Verification items for the finished model (mm, model axes). Face numbers are marked on the shaded views. Give positions to 0.01 mm unless a question says otherwise; leave off trailing zeros. Order: outer loops, then holes, each group sorted by start corner. A loop starts at its lowest first (then second) coordinate and runs counter-clockwise, first axis right, second up. Notation, with made-up numbers: (-20, 63.5) - (0, 63.5) arc R8 ccw to (0, 72.5) - close; hole circle Ø8 at (32.25, 38.5). An arc over 180 degrees is marked (long way). Answer as a JSON object with one key per item and string values.
```python
from build123d import *

# Parameters (mm, degrees)
SKETCH_1_R      = 30
EXTRUDE_1_DEPTH = 32
FILLET_1_R      = 10
SKETCH_2_R      = 5
EXTRUDE_2_DEPTH = 12


with BuildPart() as part:
    # Эскиз1 → Бобышка-Вытянуть1 (new body)
    with BuildSketch(Plane.XY):
        Circle(SKETCH_1_R)
    extrude(amount=EXTRUDE_1_DEPTH)

    # Скругление1
    fillet_1_edges = [part.edges().sort_by_distance(p)[0] for p in [
        (-30, 0, 0),
        (-30, 0, 32),
    ]]
    fillet(fillet_1_edges, radius=FILLET_1_R)

    # Эскиз2 → Бобышка-Вытянуть2 (add)
    with BuildSketch(Plane(origin=(0, 0, 0), x_dir=(-1, 0, 0), z_dir=(0, 0, -1))):
        with Locations(Location((0, 0, 0), (0, 0, 180))):
            Circle(SKETCH_2_R)
        with BuildLine():
            Line((-1.198957881, 2.75), (1.198957881, 2.75))
            ThreePointArc((1.198957881, 2.75), (3, 0), (1.198957881, -2.75))
            Line((1.198957881, -2.75), (-1.198957881, -2.75))
            ThreePointArc((-1.198957881, -2.75), (-3, 0), (-1.198957881, 2.75))
        make_face(mode=Mode.SUBTRACT)
    extrude(amount=EXTRUDE_2_DEPTH)


solid = part.part
```
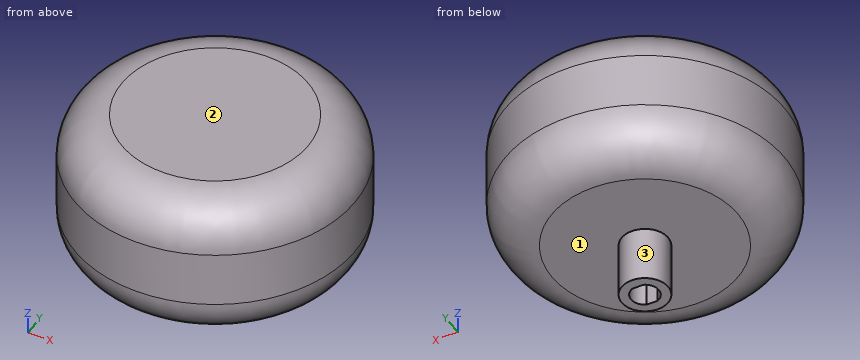
(1) Gauge pin test, flat ends, axial feed: pin 1 Ø1.2 at (x, z) = (-0.5, -4) entering from +Y; pin 2 Ø1 at (y, z) = (17.5, 7) entering from -X; pin 3 Ø6 at (y, z) = (22, 1) entering from +X. Record the tip position at first contact, or that the pin passes through.
Computed values:
{"pin 1": "stops at y = 5", "pin 2": "stops at x = -24.2", "pin 3": "stops at x = 18.68"}
(2) Section check A-A (y = 0). Record the cut outline in (x, z).
Computed values:
{"outline": "(-30, 10) arc R10 ccw to (-20, 0) - (-5, 0) - (-5, -12) - (-3, -12) - (-3, 0) - (3, 0) - (3, -12) - (5, -12) - (5, 0) - (20, 0) arc R10 ccw to (30, 10) - (30, 22) arc R10 ccw to (20, 32) - (-20, 32) arc R10 ccw to (-30, 22) - close"}
(3) Section check C-C (z = 4). Record the cut outline in (x, y).
Computed values:
{"outline": "circle Ø56 at (0, 0)"}
(4) Section check D-D (z = 9). Record the cut outline in (x, y).
Computed values:
{"outline": "circle Ø59.9 at (0, 0)"}
(5) Section check B-B (x = 0). Record the cut outline in (y, z), then the cut area to 3 significant figures.
Computed values:
{"outline": "(-30, 10) arc R10 ccw to (-20, 0) - (-5, 0) - (-5, -12) - (-2.75, -12) - (-2.75, 0) - (2.75, 0) - (2.75, -12) - (5, -12) - (5, 0) - (20, 0) arc R10 ccw to (30, 10) - (30, 22) arc R10 ccw to (20, 32) - (-20, 32) arc R10 ccw to (-30, 22) - close", "area": "1,890 mm²"}
(6) Release check for a two-part mould opening along Z. For the marked faces 1, 2 and 3 record: pulls with the +Z half, pulls with the -Z half, needs draft (parallel to the pull), parting line crosses it, or undercut.
Computed values:
{"face 1": "pulls with the -Z half", "face 2": "pulls with the +Z half", "face 3": "needs draft"}
(7) Material ranges on line 1 along Y through (x, z) = (0, -8); line 2 along Z through (x, y) = (18, -6); line 3 along Y through (x, z) = (-4, -2), recorded low to high. Write a range as [from, to].
Computed values:
{"line 1": "y = [-5, -2.75], [2.75, 5]", "line 2": "z = [0, 32]", "line 3": "y = [-3, 3]"}
